from build123d import *

# Parameters (mm, degrees)
F1_DEPTH  = 23.2
F6_DEPTH  = 12
F7_R      = 14.5
F8_DEPTH  = 38
F9_R      = 5
F10_DEPTH = 3
F9_W      = 0.8
F9_H      = 3.5
F11_DEPTH = 5
F12_R     = 1.74999
F14_R     = 1.65
F15_DEPTH = 7
F14_W     = 2
F14_H     = 10
F16_DEPTH = 20
F17_DEPTH = 7
F19_DEPTH = 10


# Not quite as in the source:
# - a fillet or chamfer is up to 0.001 mm smaller than in the source, because OpenCascade refuses the exact size


with BuildPart() as f1:
    # F0 (on Front) → F1 (new body)
    with BuildSketch(Plane.XZ):
        with BuildLine():
            ThreePointArc((16.315863747, -2.4581680554), (16.4539015408, -1.2325275198), (16.5, 0))
            ThreePointArc((16.5, 0), (16.4539015408, 1.2325275198), (16.315863747, 2.4581680554))
            ThreePointArc((16.315863747, 2.4581680554), (16.0653724653, 3.7621546421), (15.710839713, 5.0417770192))
            ThreePointArc((15.710839713, 5.0417770192), (13.1486562552, 6.8777586565), (13.1018809709, 10.0294922616))
            ThreePointArc((13.1018809709, 10.0294922616), (12.2529923089, 11.0505284706), (11.3247516529, 12))
            Line((11.3247516529, 12), (-11.3247516529, 12))
            ThreePointArc((-11.3247516529, 12), (-12.2529923089, 11.0505284706), (-13.1018809709, 10.0294922616))
            ThreePointArc((-13.1018809709, 10.0294922616), (-12.8391044723, 9.2847239636), (-12.75, 8.5))
            ThreePointArc((-12.75, 8.5), (-13.5913291851, 6.2237158574), (-15.710839713, 5.0417770192))
            ThreePointArc((-15.710839713, 5.0417770192), (-16.0653724653, 3.7621546421), (-16.315863747, 2.4581680554))
            ThreePointArc((-16.315863747, 2.4581680554), (-16.5, 0), (-16.315863747, -2.4581680554))
            ThreePointArc((-16.315863747, -2.4581680554), (-16.0653724653, -3.7621546421), (-15.710839713, -5.0417770192))
            ThreePointArc((-15.710839713, -5.0417770192), (-13.5913291851, -6.2237158574), (-12.75, -8.5))
            ThreePointArc((-12.75, -8.5), (-12.8391044723, -9.2847239636), (-13.1018809709, -10.0294922616))
            ThreePointArc((-13.1018809709, -10.0294922616), (-12.2529923089, -11.0505284706), (-11.3247516529, -12))
            Line((-11.3247516529, -12), (11.3247516529, -12))
            ThreePointArc((11.3247516529, -12), (12.2529923089, -11.0505284706), (13.1018809709, -10.0294922616))
            ThreePointArc((13.1018809709, -10.0294922616), (13.1486562552, -6.8777586566), (15.710839713, -5.0417770192))
            ThreePointArc((15.710839713, -5.0417770192), (16.0653724653, -3.7621546421), (16.315863747, -2.4581680554))
        make_face()
        with BuildLine():
            ThreePointArc((11.3247516529, 12), (12.2529923089, 11.0505284706), (13.1018809709, 10.0294922616))
            ThreePointArc((13.1018809709, 10.0294922616), (14.3930162784, 11.4667509936), (16.25, 12))
            Line((16.25, 12), (11.3247516529, 12))
        make_face()
        with BuildLine():
            ThreePointArc((-12.75, 8.5), (-12.8391044723, 9.2847239636), (-13.1018809709, 10.0294922616))
            ThreePointArc((-13.1018809709, 10.0294922616), (-14.6206205113, 7.6477091905), (-15.710839713, 5.0417770192))
            ThreePointArc((-15.710839713, 5.0417770192), (-13.5913291851, 6.2237158574), (-12.75, 8.5))
        make_face()
        with BuildLine():
            ThreePointArc((-15.710839713, 5.0417770192), (-14.6206205113, 7.6477091905), (-13.1018809709, 10.0294922616))
            ThreePointArc((-13.1018809709, 10.0294922616), (-14.3930162784, 11.4667509936), (-16.25, 12))
            ThreePointArc((-16.25, 12), (-19.3513437448, 10.1222413434), (-19.1249303104, 6.5038097008))
            ThreePointArc((-19.1249303104, 6.5038097008), (-17.627802704, 5.2826004741), (-15.710839713, 5.0417770192))
        make_face()
        with BuildLine():
            Line((-16.25, -12), (-11.3247516529, -12))
            ThreePointArc((-11.3247516529, -12), (-12.2529923089, -11.0505284706), (-13.1018809709, -10.0294922616))
            ThreePointArc((-13.1018809709, -10.0294922616), (-14.3930162784, -11.4667509936), (-16.25, -12))
        make_face()
        with BuildLine():
            Line((-11.3247516529, 12), (11.3247516529, 12))
            ThreePointArc((11.3247516529, 12), (0, 16.5), (-11.3247516529, 12))
        make_face()
        with BuildLine():
            Line((19.1249303104, -6.5038097008), (16.315863747, -2.4581680554))
            ThreePointArc((16.315863747, -2.4581680554), (16.0653724653, -3.7621546421), (15.710839713, -5.0417770192))
            ThreePointArc((15.710839713, -5.0417770192), (17.627802704, -5.2826004741), (19.1249303104, -6.5038097008))
        make_face()
        with BuildLine():
            ThreePointArc((13.1018809709, 10.0294922616), (14.6206205113, 7.6477091905), (15.710839713, 5.0417770192))
            ThreePointArc((15.710839713, 5.0417770192), (17.627802704, 5.2826004741), (19.1249303104, 6.5038097008))
            ThreePointArc((19.1249303104, 6.5038097008), (19.5900790474, 7.4541166619), (19.75, 8.5))
            ThreePointArc((19.75, 8.5), (18.7248737342, 10.9748737342), (16.25, 12))
            ThreePointArc((16.25, 12), (14.3930162784, 11.4667509936), (13.1018809709, 10.0294922616))
        make_face()
        with BuildLine():
            ThreePointArc((-16.25, -12), (-14.3930162784, -11.4667509936), (-13.1018809709, -10.0294922616))
            ThreePointArc((-13.1018809709, -10.0294922616), (-14.6206205113, -7.6477091905), (-15.710839713, -5.0417770192))
            ThreePointArc((-15.710839713, -5.0417770192), (-17.627802704, -5.2826004741), (-19.1249303104, -6.5038097008))
            ThreePointArc((-19.1249303104, -6.5038097008), (-19.3513437448, -10.1222413434), (-16.25, -12))
        make_face()
        with BuildLine():
            ThreePointArc((16.25, -12), (14.3930162784, -11.4667509936), (13.1018809709, -10.0294922616))
            ThreePointArc((13.1018809709, -10.0294922616), (12.2529923089, -11.0505284706), (11.3247516529, -12))
            Line((11.3247516529, -12), (16.25, -12))
        make_face()
        with BuildLine():
            ThreePointArc((19.1249303104, -6.5038097008), (17.627802704, -5.2826004741), (15.710839713, -5.0417770192))
            ThreePointArc((15.710839713, -5.0417770192), (14.6206205113, -7.6477091905), (13.1018809709, -10.0294922616))
            ThreePointArc((13.1018809709, -10.0294922616), (14.3930162784, -11.4667509936), (16.25, -12))
            ThreePointArc((16.25, -12), (18.7248737342, -10.9748737342), (19.75, -8.5))
            ThreePointArc((19.75, -8.5), (19.5900790474, -7.4541166619), (19.1249303104, -6.5038097008))
        make_face()
        with BuildLine():
            ThreePointArc((-13.1018809709, 10.0294922616), (-12.2529923089, 11.0505284706), (-11.3247516529, 12))
            Line((-11.3247516529, 12), (-16.25, 12))
            ThreePointArc((-16.25, 12), (-14.3930162784, 11.4667509936), (-13.1018809709, 10.0294922616))
        make_face()
        with BuildLine():
            ThreePointArc((15.710839713, 5.0417770192), (16.0653724653, 3.7621546421), (16.315863747, 2.4581680554))
            Line((16.315863747, 2.4581680554), (19.1249303104, 6.5038097008))
            ThreePointArc((19.1249303104, 6.5038097008), (17.627802704, 5.2826004741), (15.710839713, 5.0417770192))
        make_face()
        with BuildLine():
            ThreePointArc((13.1018809709, 10.0294922616), (13.1486562552, 6.8777586565), (15.710839713, 5.0417770192))
            ThreePointArc((15.710839713, 5.0417770192), (14.6206205113, 7.6477091905), (13.1018809709, 10.0294922616))
        make_face()
        with BuildLine():
            ThreePointArc((13.1018809709, -10.0294922616), (14.6206205113, -7.6477091905), (15.710839713, -5.0417770192))
            ThreePointArc((15.710839713, -5.0417770192), (13.1486562552, -6.8777586566), (13.1018809709, -10.0294922616))
        make_face()
        with BuildLine():
            ThreePointArc((-19.1249303104, -6.5038097008), (-17.627802704, -5.2826004741), (-15.710839713, -5.0417770192))
            ThreePointArc((-15.710839713, -5.0417770192), (-16.0653724653, -3.7621546421), (-16.315863747, -2.4581680554))
            Line((-16.315863747, -2.4581680554), (-19.1249303104, -6.5038097008))
        make_face()
        with BuildLine():
            ThreePointArc((-15.710839713, -5.0417770192), (-14.6206205113, -7.6477091905), (-13.1018809709, -10.0294922616))
            ThreePointArc((-13.1018809709, -10.0294922616), (-12.8391044723, -9.2847239636), (-12.75, -8.5))
            ThreePointArc((-12.75, -8.5), (-13.5913291851, -6.2237158574), (-15.710839713, -5.0417770192))
        make_face()
        with BuildLine():
            ThreePointArc((-16.315863747, 2.4581680554), (-16.0653724653, 3.7621546421), (-15.710839713, 5.0417770192))
            ThreePointArc((-15.710839713, 5.0417770192), (-17.627802704, 5.2826004741), (-19.1249303104, 6.5038097008))
            Line((-19.1249303104, 6.5038097008), (-16.315863747, 2.4581680554))
        make_face()
        with BuildLine():
            ThreePointArc((-11.3247516529, -12), (0, -16.5), (11.3247516529, -12))
            Line((11.3247516529, -12), (-11.3247516529, -12))
        make_face()
    extrude(amount=-F1_DEPTH)

    # F2 (on Right) → F3 (revolve)
    with BuildSketch(Plane.YZ):
        Polygon((0, 14.4998934947), (0, 16.1), (-13, 15.95), (-12.9815396904, 14.3501064982), align=None)
    revolve(axis=Axis((0, -6.5, 11.45), (0, -1, 0)))

    # F2 (on Right) → F4 (revolve)
    with BuildSketch(Plane.YZ):
        Polygon((0, -1.5001065053), (0, 0.1), (-13, -0.05), (-12.9815396904, -1.6498935018), align=None)
    revolve(axis=Axis((0, -6.5, -4.55), (0, -1, 0)))

    # F5 (on face) → F6 (join)
    with BuildSketch(Plane(origin=(0, 23.2, 0), x_dir=(-1, 0, 0), z_dir=(0, 1, 0))):
        with BuildLine():
            ThreePointArc((16.315863747, -2.4581680554), (16.4539015408, -1.2325275198), (16.5, 0))
            ThreePointArc((16.5, 0), (16.4539015408, 1.2325275198), (16.315863747, 2.4581680554))
            ThreePointArc((16.315863747, 2.4581680554), (14.6206205113, 7.6477091906), (11.3247516529, 12))
            ThreePointArc((11.3247516529, 12), (0, 16.5), (-11.3247516529, 12))
            ThreePointArc((-11.3247516529, 12), (-14.6206205113, 7.6477091906), (-16.315863747, 2.4581680554))
            ThreePointArc((-16.315863747, 2.4581680554), (-16.5, 0), (-16.315863747, -2.4581680554))
            ThreePointArc((-16.315863747, -2.4581680554), (-14.6206205113, -7.6477091905), (-11.3247516529, -12))
            ThreePointArc((-11.3247516529, -12), (0, -16.5), (11.3247516529, -12))
            ThreePointArc((11.3247516529, -12), (14.6206205113, -7.6477091906), (16.315863747, -2.4581680554))
        make_face()
    extrude(amount=F6_DEPTH)

    # F7 (on face) → F8 (join)
    with BuildSketch(Plane(origin=(0, 35.2, 0), x_dir=(-1, 0, 0), z_dir=(0, 1, 0))):
        Circle(F7_R)
    extrude(amount=F8_DEPTH)

    # F9 (on face) → F10 (join)
    with BuildSketch(Plane(origin=(0, 73.2, 0), x_dir=(-1, 0, 0), z_dir=(0, 1, 0))):
        Circle(F9_R)
    extrude(amount=F10_DEPTH)

    # F9 (on face) → F11 (join)
    with BuildSketch(Plane(origin=(0, 73.2, 0), x_dir=(-1, 0, 0), z_dir=(0, 1, 0))):
        with Locations((-10.6, 0)):
            Rectangle(F9_W, F9_H)
        with Locations((10.6, 0)):
            Rectangle(F9_W, F9_H)
    extrude(amount=F11_DEPTH)

    # F12 (radius 1.75 in the source; OpenCascade refuses exactly that, so slightly less here)
    f12_edges = [f1.edges().sort_by_distance(p)[0] for p in [
        (-10.6, 78.2, -1.75),
        (-10.6, 78.2, 1.75),
        (10.6, 78.2, -1.75),
        (10.6, 78.2, 1.75),
    ]]
    fillet(f12_edges, radius=F12_R)

    # F14 (on offset) → F15 (join)
    with BuildSketch(Plane.XY.offset(-20)):
        with BuildLine():
            ThreePointArc((-25, 20.2), (-30, 15.2), (-25, 10.2))
            Line((-25, 10.2), (25, 10.2))
            ThreePointArc((25, 10.2), (30, 15.2), (25, 20.2))
            Line((25, 20.2), (-25, 20.2))
        make_face()
        with Locations((-25, 15.2)):
            Circle(F14_R, mode=Mode.SUBTRACT)
        with Locations((25, 15.2)):
            Circle(F14_R, mode=Mode.SUBTRACT)
    extrude(amount=F15_DEPTH)

    # F14 (on offset) → F16 (join)
    with BuildSketch(Plane.XY.offset(-20)):
        with Locations((-14, 65.2)):
            Rectangle(F14_W, F14_H)
        with Locations((14, 65.2)):
            Rectangle(F14_W, F14_H)
    extrude(amount=F16_DEPTH)

    # F14 (on offset) → F17 (join)
    with BuildSketch(Plane.XY.offset(-20)):
        with BuildLine():
            ThreePointArc((-25, 70.2), (-30, 65.2), (-25, 60.2))
            Line((-25, 60.2), (-15, 60.2))
            Line((-15, 60.2), (-15, 70.2))
            Line((-15, 70.2), (-25, 70.2))
        make_face()
        with Locations((-25, 65.2)):
            Circle(F14_R, mode=Mode.SUBTRACT)
        with BuildLine():
            Line((15, 70.2), (15, 60.2))
            Line((15, 60.2), (25, 60.2))
            ThreePointArc((25, 60.2), (30, 65.2), (25, 70.2))
            Line((25, 70.2), (15, 70.2))
        make_face()
        with Locations((25, 65.2)):
            Circle(F14_R, mode=Mode.SUBTRACT)
    extrude(amount=F17_DEPTH)

    # F18 (on face) → F19 (join, through all)
    with BuildSketch(Plane(origin=(0, 70.2, 0), x_dir=(-1, 0, 0), z_dir=(0, 1, 0))):
        with BuildLine():
            Line((14.5, 0), (15, 0))
            ThreePointArc((15, 0), (-14.4913767462, 3.8729833462), (13, -7.4833147735))
            Line((13, -7.4833147735), (13, -6.4226162893))
            ThreePointArc((13, -6.4226162893), (14.1200212464, -3.2977264896), (14.5, 0))
        make_face()
    extrude(amount=-F19_DEPTH)


solid = f1.part
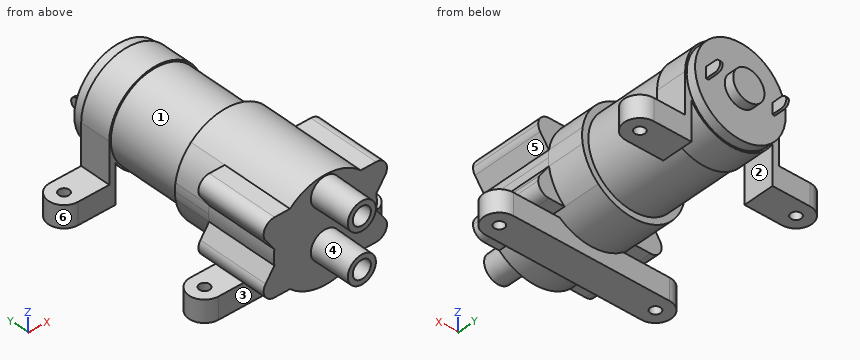
Geometry check sheet. Reference: the model listing, model coordinates, mm. Face numbers are marked on the shaded views. A direction names the side the tool comes from. Round coordinates to 2 decimals unless told otherwise and drop trailing zeros. Order: outer loops, then holes, each group sorted by start corner. A loop starts at its lowest first (then second) coordinate and runs counter-clockwise, first axis right, second up. Notation, with made-up numbers: (-28, 9.25) - (11, 9.25) arc R28 cw to (11, 27.25) - close; hole circle Ø2 at (-13.75, 52.25). An arc over 180 degrees is marked (long way). One line per question, with ' | ' between items. Start each with the question number.
(1) Sectioned sample at B-B on y = 27.5. Record the cut outline in (x, z), and give its area (3 significant figures).
(2) Sectioned sample at A-A on y = 65.2. Record the cut outline in (x, z), and give its area (3 significant figures).
(3) Thickness scan on L1, parallel to Y at x = 25, z = -16.5; L2, parallel to X at y = 65.2, z = -17; L3, parallel to Z at x = 13.5, y = 15. Record the ranges inside material, lowest first. Write a range as [from, to].
(4) Access from +Z, -Z, +X, -X, +Y, -Y to the whole of each face (thin tool, end or side, straight path). Record for the marked faces 1, 2 and 3.
(5) Depth check by flat-ended pin: pin 1 Ø6 at (y, z) = (31, -1) entering from -X; pin 2 Ø3.5 at (x, z) = (-10, -16) entering from +Y; pin 3 Ø5 at (x, y) = (-19, 65.5) entering from +Z; pin 4 Ø3 at (x, y) = (25, 65.2) entering from -Z. Enter the tip coordinate at first touch or a pass-through.
(6) Sectioned sample at C-C on y = 15.2. Count the separate pieces of the cut face and the enclosed holes in it, and give its area (3 significant figures).
(7) Sectioned sample at D-D on y = 2. Record the cut outline in (x, z), and give its area (3 significant figures).
(8) Release check for a two-part mould opening along Y. For the marked faces 4, 5 and 6 record: released by +Y, released by -Y, zero draft, split by the parting line, or undercut.
Conclusion:
1) outline: circle Ø33 at (0, 0) | area: 855 mm2
2) outline: (-30, -20) - (-26.65, -20) - (-26.65, -13) - (-30, -13) - close; (-23.35, -20) - (-13, -20) - (-13, -7.48) arc R15 ccw to (13, -7.48) - (13, -20) - (23.35, -20) - (23.35, -13) - (15, -13) - (15, 0) arc R15 ccw to (-15, 0) - (-15, -13) - (-23.35, -13) - close; (26.65, -20) - (30, -20) - (30, -13) - (26.65, -13) - close | area: 930 mm2
3) L1: y = [10.2, 13.55], [16.85, 20.2], [60.2, 63.55], [66.85, 70.2] | L2: x = [-30, -26.65], [-23.35, -13], [13, 23.35], [26.65, 30] | L3: z = [-20, -13], [-12, 12]
4) face 1: none | face 2: -Z, +Y | face 3: -Z, -Y
5) pin 1: stops at x = -16.5 | pin 2: stops at y = 20.2 | pin 3: stops at z = -13 | pin 4: passes through
6) separate pieces: 3 | enclosed holes: 0 | area: 1,340 mm2
7) outline: (-19.12, -6.5) arc R3.5 ccw to (-16.25, -12) - (-11.32, -12) arc R16.5 ccw to (11.32, -12) - (16.25, -12) arc R3.5 ccw to (19.12, -6.5) - (16.32, -2.46) arc R16.5 ccw to (16.32, 2.46) - (19.12, 6.5) arc R3.5 ccw to (16.25, 12) - (11.32, 12) arc R16.5 ccw to (-11.32, 12) - (-16.25, 12) arc R3.5 ccw to (-19.12, 6.5) - (-16.32, 2.46) arc R16.5 ccw to (-16.32, -2.46) - close | area: 1,010 mm2
8) face 4: released by -Y | face 5: zero draft | face 6: undercut
